Geometry: final body of the model. Coordinates: model frame, mm. A direction names the side the tool comes from. Give positions to 0.01 mm unless a question says otherwise; leave off trailing zeros. Order: outer loops, then holes, each group sorted by start corner. A loop starts at its lowest first (then second) coordinate and runs counter-clockwise, first axis right, second up. Notation, with made-up numbers: (-5.5, -26.5) -> (43.5, -26.5) arc R16 cw to (43.5, -1.5) -> close; hole circle Ø3 at (72, 30). An arc over 180 degrees is marked (long way). Answer in a Markdown table with one row per item. Add a question column.
Q1. Cut plane D-D on x = -599.5. Return the cut outline in (y, z), and give its area (3 significant figures).
Q2. Pull-direction query (X, two-part tool) for faces 1 (the face through (-626, -2, 10)), 2 (the face through (-595.009, -2, 7)), 3 (the face through (-614.009, 16, 0)); classes: +X half, -X half, draft (parallel to the pull), parting line (faces both ways), or undercut.
Q3. Set-up query: faces 4 (the face through (-612.009, -3, 0)), 5 (the face through (-607.509, 18, 0)), 6 (the face through (-613, 17, 0)), 7 (the face through (-648.495, -1.884, -4.084)). Return all of +Z, -Z, +X, -X, +Y, -Y with unobstructed straight access to the full face (end or side cutting, diameter ignored); none if empty.
Q4. Cut plane B-B on y = -2.5. Return the cut outline in (x, z), and give its area (3 significant figures).
Q5. Contact query for flat-ended pins moving along their axis: P1, Ø8.5, axis at x = -635, y = -3.5, coming from the -Z side; P2, Ø3.5, axis at y = -2, z = -1, coming from the +X side; P3, Ø1.5, axis at x = -648, z = 3.5, coming from the +Y side; P4, Ø6.5, axis at x = -609.5, z = 3, coming from the +Y side. Output: stop coordinate, or through.
Q6. Cut plane C-C on z = 8.75. Return the cut outline in (x, y), and give its area (3 significant figures).
Q7. Line query: line 1 along Y through (x, z) = (-613.5, -3.25); line 2 along Z through (x, y) = (-630, -13); line 3 along X through (y, z) = (3.5, 2.25). Output: solid intervals per line, ascending. Write a range as from..to.
Q8. Cut plane A-A on z = 0. Return the cut outline in (x, y).
from build123d import *

# Parameters (mm, degrees)
ESQUISSE1_R                  = 7.5
BOSS_EXTRU_1_DEPTH           = 10
ESQUISSE1_3_W                = 17
ESQUISSE1_3_H                = 6
ENL_V_MAT_EXTRU_1_DEPTH      = 2
ENL_V_MAT_EXTRU_1_DEPTH_BACK = 10
ESQUISSE1_5_R                = 14
ENL_V_MAT_EXTRU_2_DEPTH      = 658.559578744
ENL_V_MAT_EXTRU_2_DEPTH_BACK = 658.559578744
ESQUISSE1_6_R                = 2
ENL_V_MAT_EXTRU_3_DEPTH      = 658.559578745
ENL_V_MAT_EXTRU_3_DEPTH_BACK = 658.559578745


with BuildPart() as part:
    # Esquisse1 → Boss.-Extru.1 (new, symmetric)
    with BuildSketch(Plane.XY):
        with BuildLine():
            Line((-634.508066615, 20), (-595.008671928, 20))
            Line((-595.008671928, 20), (-595.008671928, -25))
            Line((-595.008671928, -25), (-634.508066615, -25))
            ThreePointArc((-634.508066615, -25), (-657.008066615, -2.5), (-634.508066615, 20))
        make_face()
        with Locations((-634.508066615, -2.5)):
            Circle(ESQUISSE1_R, mode=Mode.SUBTRACT)
    extrude(amount=BOSS_EXTRU_1_DEPTH, both=True)

    # Esquisse1_3 → Enl_vement de mati_re-R_volution1 (revolve, cut)
    with BuildSketch(Plane.XY, mode=Mode.PRIVATE) as enl_vement_de_mati_re_r_volution1_sk:
        with Locations((-603.508671928, 0.5)):
            Rectangle(ESQUISSE1_3_W, ESQUISSE1_3_H)
    revolve(enl_vement_de_mati_re_r_volution1_sk.sketch.rotate(Axis((-666.113025571, -2.5, 0), (1, 0, 0)), 90), axis=Axis((-666.113025571, -2.5, 0), (1, 0, 0)), mode=Mode.SUBTRACT)

    # Esquisse1_5 → Enl_v. mat.-Extru.1 (cut, two sides: drawn at the far end of the back side and taken through both)
    with BuildSketch(Plane.XY.offset(-ENL_V_MAT_EXTRU_1_DEPTH_BACK)):
        with Locations((-634.508066615, -2.5)):
            Circle(ESQUISSE1_5_R)
    extrude(amount=ENL_V_MAT_EXTRU_1_DEPTH + ENL_V_MAT_EXTRU_1_DEPTH_BACK, mode=Mode.SUBTRACT)

    # Esquisse1_6 → Enl_v. mat.-Extru.2 (cut, two sides: drawn at the far end of the back side and taken through both)
    with BuildSketch(Plane.XY.offset(-ENL_V_MAT_EXTRU_2_DEPTH_BACK)):
        with Locations((-604.008671928, 3.5)):
            Circle(ESQUISSE1_6_R)
    extrude(amount=ENL_V_MAT_EXTRU_2_DEPTH + ENL_V_MAT_EXTRU_2_DEPTH_BACK, mode=Mode.SUBTRACT)

    # Esquisse1_7 → Enl_v. mat.-Extru.3 (cut, two sides: drawn at the far end of the back side and taken through both)
    with BuildSketch(Plane.XY.offset(-ENL_V_MAT_EXTRU_3_DEPTH_BACK)):
        Polygon((-607.508671928, 20), (-612.508671928, 20), (-612.508671928, 17), (-614.008671928, 17), (-614.008671928, 14), (-606.008671928, 14), (-606.008671928, 17), (-607.508671928, 17), align=None)
    extrude(amount=ENL_V_MAT_EXTRU_3_DEPTH + ENL_V_MAT_EXTRU_3_DEPTH_BACK, mode=Mode.SUBTRACT)


solid = part.part
Completed:
| question | item | result |
|---|---|---|
| 1 | outline | (-25, -10) -> (20, -10) -> (20, 10) -> (-25, 10) -> close; hole circle Ø12 at (-2.5, 0) |
| 1 | area | 787 mm² |
| 2 | face 1 | draft |
| 2 | face 2 | +X half |
| 2 | face 3 | undercut |
| 3 | face 4 | +X |
| 3 | face 5 | +Z, -Z, +Y |
| 3 | face 6 | +Z, -Z |
| 3 | face 7 | -Z |
| 4 | outline | (-657.01, -10) -> (-648.51, -10) -> (-648.51, 2) -> (-642.01, 2) -> (-642.01, 10) -> (-657.01, 10) -> close; (-627.01, 2) -> (-620.51, 2) -> (-620.51, -10) -> (-595.01, -10) -> (-595.01, -6) -> (-612.01, -6) -> (-612.01, 6) -> (-595.01, 6) -> (-595.01, 10) -> (-627.01, 10) -> close |
| 4 | area | 580 mm² |
| 5 | P1 | passes through |
| 5 | P2 | stops at x = -612.01 |
| 5 | P3 | stops at y = 16.04 |
| 5 | P4 | stops at y = 20 |
| 6 | outline | (-634.51, -25) -> (-595.01, -25) -> (-595.01, 20) -> (-607.51, 20) -> (-607.51, 17) -> (-606.01, 17) -> (-606.01, 14) -> (-614.01, 14) -> (-614.01, 17) -> (-612.51, 17) -> (-612.51, 20) -> (-634.51, 20) arc R22.5 ccw to start; hole circle Ø15 at (-634.51, -2.5); hole circle Ø4 at (-604.01, 3.5) |
| 6 | area | 2,340 mm² |
| 7 | line 1 | y = -25..14, 17..20 |
| 7 | line 2 | z = 2..10 |
| 7 | line 3 | x = -656.19..-639.01, -630.01..-606.01, -602.01..-595.01 |
| 8 | outline | (-634.51, -25) -> (-595.01, -25) -> (-595.01, -8.5) -> (-612.01, -8.5) -> (-612.01, 3.5) -> (-606.01, 3.5) arc R2 cw to (-602.01, 3.5) -> (-595.01, 3.5) -> (-595.01, 20) -> (-607.51, 20) -> (-607.51, 17) -> (-606.01, 17) -> (-606.01, 14) -> (-614.01, 14) -> (-614.01, 17) -> (-612.51, 17) -> (-612.51, 20) -> (-634.51, 20) arc R22.5 ccw to start; hole circle Ø28 at (-634.51, -2.5) |
